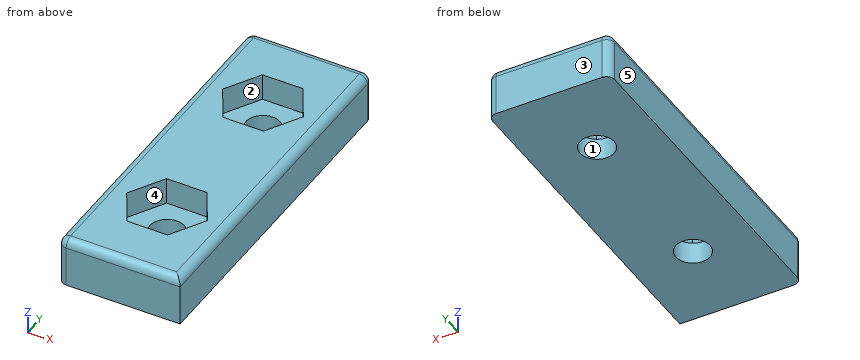
from build123d import *

# Parameters (mm, degrees)
F0_W     = 15
F0_H     = 42
F0_R     = 2.1
F1_DEPTH = 6
F2_DEPTH = 6.001
F3_R     = 2.1
F4_DEPTH = 3.3
F5_R     = 1


# Not quite as in the source:
# - a feature names something its author has since deleted; it is built from what else it names


with BuildPart() as f1:
    # F0 (on Top) → F1 (new body)
    with BuildSketch(Plane.XY):
        Rectangle(F0_W, F0_H)
        with Locations((0, -10.5)):
            Circle(F0_R, mode=Mode.SUBTRACT)
        with Locations((0, 10.5)):
            Circle(F0_R, mode=Mode.SUBTRACT)
        with Locations((0, -10.5)):
            Circle(F0_R)
        with Locations((0, 10.5)):
            Circle(F0_R)
    extrude(amount=F1_DEPTH)

    # F0 (on Top) → F2 (cut, through all)
    with BuildSketch(Plane.XY):
        with Locations((0, 10.5)):
            Circle(F0_R)
        with Locations((0, -10.5)):
            Circle(F0_R)
    extrude(amount=F2_DEPTH, mode=Mode.SUBTRACT)

    # F3 (on face) → F4 (cut)
    with BuildSketch(Plane.XY.offset(6)):
        Polygon((4.965212315, -10.5), (2.4826061575, -6.2), (-2.4826061575, -6.2), (-4.965212315, -10.5), (-2.4826061575, -14.8), (2.4826061575, -14.8), align=None)
        with Locations((0, -10.5)):
            Circle(F3_R, mode=Mode.SUBTRACT)
        Polygon((4.965212315, 10.5), (2.4826061575, 14.8), (-2.4826061575, 14.8), (-4.965212315, 10.5), (-2.4826061575, 6.2), (2.4826061575, 6.2), align=None)
        with Locations((0, 10.5)):
            Circle(F3_R, mode=Mode.SUBTRACT)
    extrude(amount=-F4_DEPTH, mode=Mode.SUBTRACT)

    # F5
    f5_edges = [f1.edges().sort_by_distance(p)[0] for p in [
        (-7.5, 21, 3),
        (-7.5, -21, 3),
        (0, -21, 6),
        (-7.5, 0, 6),
        (0, 21, 6),
        (7.5, 0, 6),
        (7.5, 21, 3),
    ]]
    fillet(f5_edges, radius=F5_R)


solid = f1.part
Geometry check sheet. Reference: the model listing, model coordinates, mm. Face numbers are marked on the shaded views. A direction names the side the tool comes from. Give positions to 0.01 mm unless a question says otherwise; leave off trailing zeros. Loops run counter-clockwise (first coordinate to the right, second up) from the corner with the lowest first, then second, coordinate; pieces in that order, holes last.
(1) Set-up check for the marked faces 1 and 2: record each of +Z, -Z, +X, -X, +Y, -Y from which the full face is reachable in a straight line by a thin tool's end or side.
From the geometry:
face 1: +Z, -Z
face 2: +Z
(2) Section check D-D on x = -4.5. Record the cut outline in (y, z).
From the geometry:
outline: (-21, 0) - (21, 0) - (21, 5) arc R1 ccw to (20, 6) - (11.31, 6) - (11.31, 2.7) - (9.69, 2.7) - (9.69, 6) - (-9.69, 6) - (-9.69, 2.7) - (-11.31, 2.7) - (-11.31, 6) - (-20, 6) arc R1 ccw to (-21, 5) - close
(3) Release check for a two-part mould opening along Y. For the marked faces 3, 4 and 5 record: released by +Y, released by -Y, zero draft, split by the parting line, or undercut.
From the geometry:
face 3: released by +Y
face 4: undercut
face 5: zero draft
(4) Section check C-C on y = -11. Record the cut outline in (x, z).
From the geometry:
outline: (-7.5, 0) - (-2.04, 0) - (-2.04, 2.7) - (-4.68, 2.7) - (-4.68, 6) - (-6.5, 6) arc R1 ccw to (-7.5, 5) - close; (2.04, 0) - (7.5, 0) - (7.5, 5) arc R1 ccw to (6.5, 6) - (4.68, 6) - (4.68, 2.7) - (2.04, 2.7) - close
(5) Depth check by flat-ended pin: pin 1 Ø6.5 at (x, y) = (0, -10.5) entering from +Z. Enter the tip coordinate at first touch or a pass-through.
From the geometry:
pin 1: stops at z = 2.7
(6) Thickness scan on L1, parallel to Y at x = 0, z = 1.5; L2, parallel to Y at x = -3.25, z = 4.4; L3, parallel to Z at x = -1.5, y = 7. Record the ranges inside material, lowest first.
From the geometry:
L1: y = -21 to -12.6, -8.4 to 8.4, 12.6 to 21
L2: y = -21 to -13.47, -7.53 to 7.53, 13.47 to 21
L3: z = 0 to 2.7
(7) Section check A-A on x = 0. Record the cut outline in (y, z).
From the geometry:
outline: (-21, 0) - (-12.6, 0) - (-12.6, 2.7) - (-14.8, 2.7) - (-14.8, 6) - (-20, 6) arc R1 ccw to (-21, 5) - close; (-8.4, 0) - (8.4, 0) - (8.4, 2.7) - (6.2, 2.7) - (6.2, 6) - (-6.2, 6) - (-6.2, 2.7) - (-8.4, 2.7) - close; (12.6, 0) - (21, 0) - (21, 5) arc R1 ccw to (20, 6) - (14.8, 6) - (14.8, 2.7) - (12.6, 2.7) - close
(8) Section check B-B on z = 2.1. Record the cut outline in (x, y).
From the geometry:
outline: (-7.5, -20) arc R1 ccw to (-6.5, -21) - (7.5, -21) - (7.5, 20) arc R1 ccw to (6.5, 21) - (-6.5, 21) arc R1 ccw to (-7.5, 20) - close; hole circle Ø4.2 at (0, -10.5); hole circle Ø4.2 at (0, 10.5)
